Source: CAD feature listing. Evaluate the final solid. Frame: model axes, mm. Face numbers are marked on the shaded views. Round coordinates to 2 decimals unless told otherwise and drop trailing zeros. Order: outer loops, then holes, each group sorted by start corner. A loop starts at its lowest first (then second) coordinate and runs counter-clockwise, first axis right, second up. Notation, with made-up numbers: (-6.75, 15.5) - (15.25, 15.5) arc R26 ccw to (15.25, 50.5) - close; hole circle Ø9 at (23, 65). An arc over 180 degrees is marked (long way). Use one line per item in the form item = value. Start each with the question number.
Q1. Cut plane A-A, the plane x = 40. Return the cut outline in (y, z), and give its area (3 significant figures).
Q2. Pin query (flat end, axial travel): pin 1 Ø2 at (x, z) = (40, 1) entering from -Y. Return the tip coordinate at first contact, or that it passes through.
Q3. Ray query, line 1 (Y direction, x = -1, z = 1.6); line 2 (Y direction, x = 30, z = 2); line 3 (Y direction, x = -2, z = 3.2). Return the intervals inside material, ascending. Write a range as [from, to].
Q4. Cut plane D-D, the plane y = -22.5. Return the cut outline in (x, z), and give its area (3 significant figures).
Q5. Cut plane C-C, the plane z = 2.85. Give the number of separate pieces and of enclosed holes in the cut face, and give its area (3 significant figures).
Q6. Cut plane B-B, the plane y = 17.12. Return the cut outline in (x, z), and give its area (3 significant figures).
Q7. Draft query along Z for the marked faces 1 and 2. Return one class per face: released by +Z, released by -Z, zero draft, split by the parting line, or undercut.
from build123d import *

# Parameters (mm, degrees)
SKETCH_1_R      = 4.25
SKETCH_1_R_2    = 8.75
SKETCH_1_R_3    = 2
SKETCH_1_R_4    = 1.25
EXTRUDE_1_DEPTH = 4


with BuildPart() as part:
    # 草图1 → 凸台-拉伸1 (new body)
    with BuildSketch(Plane.XY):
        with BuildLine():
            Line((-1, 20), (99.064295006, 20))
            ThreePointArc((99.064295006, 20), (119.064295006, 0), (99.064295006, -20))
            Line((99.064295006, -20), (10.014533743, -20))
            Line((10.014533743, -20), (3, -30))
            ThreePointArc((3, -30), (-1, -34), (-5, -30))
            Line((-5, -30), (-17.208156126, -11.717323713))
            ThreePointArc((-17.208156126, -11.717323713), (-18.809358134, 9.10092099), (-1, 20))
        make_face()
        with Locations((-1, 0)):
            Circle(SKETCH_1_R, mode=Mode.SUBTRACT)
        with Locations((99.064295006, 0)):
            Circle(SKETCH_1_R_2, mode=Mode.SUBTRACT)
        with Locations((85.534295006, 0)):
            Circle(SKETCH_1_R_3, mode=Mode.SUBTRACT)
        with Locations((105.829295006, 11.717323713)):
            Circle(SKETCH_1_R_3, mode=Mode.SUBTRACT)
        with Locations((105.829295006, -11.717323713)):
            Circle(SKETCH_1_R_3, mode=Mode.SUBTRACT)
        with Locations((-1, -30)):
            Circle(SKETCH_1_R_3, mode=Mode.SUBTRACT)
        with Locations((-1, 17.12)):
            Circle(SKETCH_1_R_4, mode=Mode.SUBTRACT)
        with BuildLine():
            Line((23.78352134, 10.95385289), (60.46647866, 10.95385289))
            ThreePointArc((60.46647866, 10.95385289), (71.420331549, 0), (60.46647866, -10.95385289))
            Line((60.46647866, -10.95385289), (23.78352134, -10.95385289))
            ThreePointArc((23.78352134, -10.95385289), (12.829668451, 0), (23.78352134, 10.95385289))
        make_face(mode=Mode.SUBTRACT)
    extrude(amount=EXTRUDE_1_DEPTH)


solid = part.part
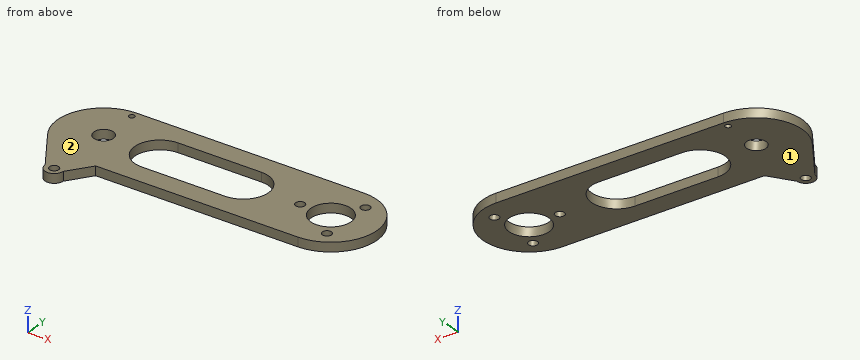
Completed:
q1.outline = (-20, 0) - (-10.95, 0) - (-10.95, 4) - (-20, 4) - close; (10.95, 0) - (20, 0) - (20, 4) - (10.95, 4) - close
q1.area = 72.4 mm2
q2.pin_1 = -20
q3.line_1 = [-34, -32], [-28, -4.25], [4.25, 15.87], [18.37, 20]
q3.line_2 = [-20, -10.95], [10.95, 20]
q3.line_3 = [-33.87, -31.73], [-28.27, -4.13], [4.13, 16.37], [17.87, 19.97]
q4.outline = (-10.01, 0) - (8.26, 0) - (8.26, 4) - (-10.01, 4) - close
q4.area = 73.1 mm2
q5.separate_pieces = 1
q5.enclosed_holes = 8
q5.area = 3,920 mm2
q6.outline = (-11.34, 0) - (-2.25, 0) - (-2.25, 4) - (-11.34, 4) - close; (0.25, 0) - (109.4, 0) - (109.4, 4) - (0.25, 4) - close
q6.area = 473 mm2
q7.face_1 = released by -Z
q7.face_2 = released by +Z
